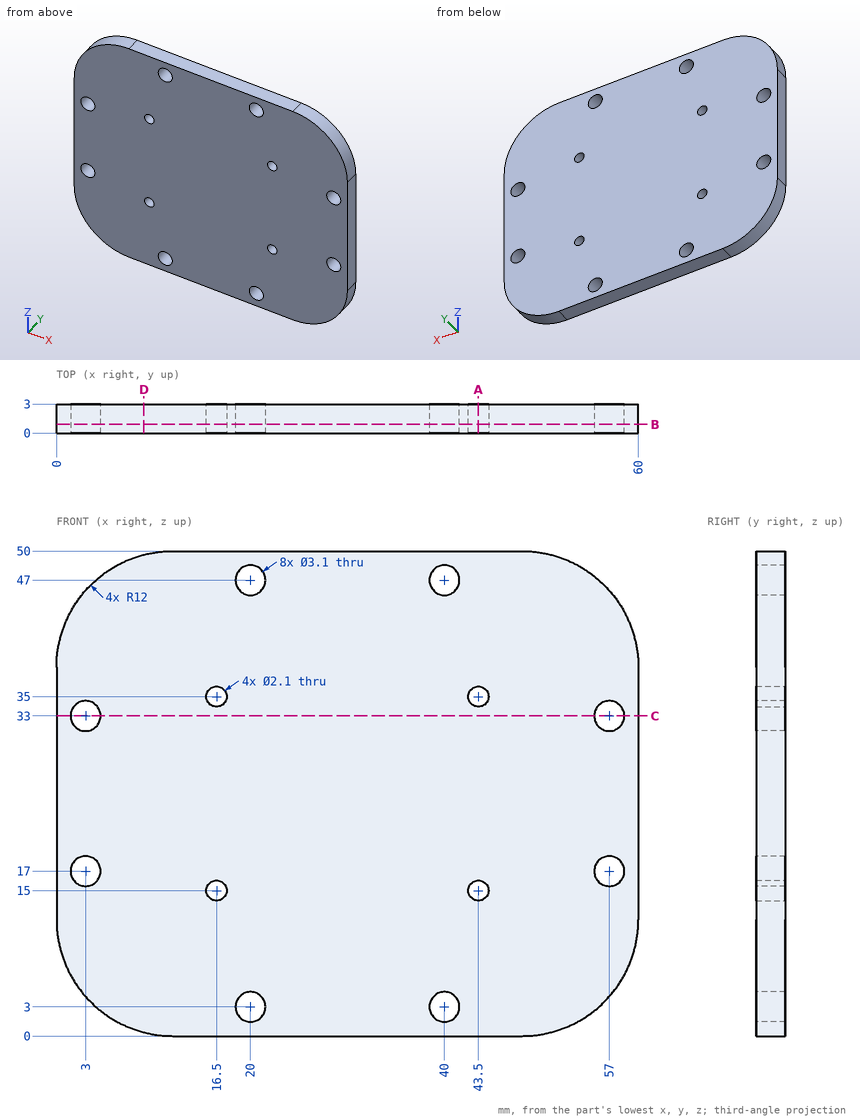
Could you check a few things on this drawing? It's one solid part, dimensions in mm from its lowest x, y, z. Round coordinates to 2 decimals unless told otherwise and drop trailing zeros. Write each loop counter-clockwise with the first axis right and the second up, starting at its lowest first coordinate (ties: lowest second). Pieces come first, ordered by that corner, then holes. Notation, with made-up numbers: M 44,-4 L 82,-4 A31 ccw 82,30 Z; hole C 61,89 d11. An arc over 180 degrees is marked long. Answer as CSV lines item,"result". Start each with the question number.
1. Suppose I cut it at B-B on y = 0.9. Count the separate pieces of the cut face and the enclosed holes in it, then the cut area to 3 significant figures.
2. I need wall thicknesses on probe 1 along Z at (x, y) = (20, 0.9); probe 2 along X at (y, z) = (2, 15); probe 3 along Z at (x, y) = (16.5, 1.6). Which ranges of each line are inside material? Lowest first, please.
3. I'm going to push flat-ended pins straight in: pin 1 Ø1.9 at (x, z) = (20, 47) entering from +Y; pin 2 Ø1 at (y, z) = (1.5, 43) entering from -X. Where does each tip first touch, or does it pass through?
4. Suppose I cut it at A-A on x = 43.5. Write out the boundary of the cut face in (y, z).
5. Suppose I cut it at D-D on x = 9. Write out the boundary of the cut face in (y, z).
6. Suppose I cut it at C-C on z = 33. Write out the boundary of the cut face in (x, y).
Check result:
1,separate pieces,"1"
1,enclosed holes,"12"
1,area,"2,800 mm2"
2,probe 1,"z = 0 to 1.45, 4.55 to 45.45, 48.55 to 50"
2,probe 2,"x = 0 to 15.45, 17.55 to 42.45, 44.55 to 60"
2,probe 3,"z = 0 to 13.95, 16.05 to 33.95, 36.05 to 50"
3,pin 1,"passes through"
3,pin 2,"stops at x = 0.88"
4,outline,"M 0,0 L 3,0 L 3,13.95 L 0,13.95 Z; M 0,16.05 L 3,16.05 L 3,33.95 L 0,33.95 Z; M 0,36.05 L 3,36.05 L 3,50 L 0,50 Z"
5,outline,"M 0,0.38 L 3,0.38 L 3,49.62 L 0,49.62 Z"
6,outline,"M 0,0 L 1.45,0 L 1.45,3 L 0,3 Z; M 4.55,0 L 55.45,0 L 55.45,3 L 4.55,3 Z; M 58.55,0 L 60,0 L 60,3 L 58.55,3 Z"
